Build history of the part. All positions in model axes, mm. A direction names the side the tool comes from. Coordinates: 2 decimals unless noted, no trailing zeros. Write each loop counter-clockwise with the first axis right and the second up, starting at its lowest first coordinate (ties: lowest second). Pieces come first, ordered by that corner, then holes.
```python
from build123d import *

# Parameters (mm, degrees)
SKETCH_1_W             = 130
SKETCH_1_H             = 130
EXTRUDE_1251_DEPTH     = 5
EXTRUDE_1478_DEPTH     = 25
SKETCH_3_R             = 17.5
CUT_EXTRUDE_1_DEPTH    = 85
SKETCH_4_R             = 17.5
CUT_EXTRUDE_2_DEPTH    = 85
SKETCH_8_W             = 52
SKETCH_8_H             = 25
CUT_EXTRUDE_1_2_DEPTH  = 10
SKETCH_9_W             = 52
SKETCH_9_H             = 25
CUT_EXTRUDE_2_2_DEPTH  = 10
SKETCH_5_W             = 2
SKETCH_5_H             = 2
SKETCH_5_H_2           = 43
SKETCH_5_W_2           = 43
EXTRUDE_2758_DEPTH     = 25
SKETCH_7_W             = 33.5
SKETCH_7_H             = 33.5
EXTRUDE_2892_DEPTH     = 13
HOLE_WIZARD_2949_D     = 5
HOLE_WIZARD_2949_DEPTH = 5
HOLE_WIZARD_2949_TIP   = 1.502151548
HOLE_WIZARD_1_D        = 2.5
HOLE_WIZARD_2_D        = 2.5
HOLE_WIZARD_6774_D     = 2.5
HOLE_WIZARD_1_2_D      = 2.5
HOLE_WIZARD_2_2_D      = 2.5


with BuildPart() as part:
    # 草图1 → Extrude 1251 (new body)
    with BuildSketch(Plane(origin=(0, 0, 0), x_dir=(1, 0, 0), z_dir=(0, 1, 0))):
        with Locations((65, 65)):
            Rectangle(SKETCH_1_W, SKETCH_1_H)
    extrude(amount=EXTRUDE_1251_DEPTH)

    # 草图2 → Extrude 1478 (add)
    with BuildSketch(Plane(origin=(0, 5, 0), x_dir=(1, 0, 0), z_dir=(0, 1, 0))):
        Polygon((0, 85), (0, 0), (52, 0), (52, 78), (130, 78), (130, 130), (45, 130), (45, 85), align=None)
    extrude(amount=EXTRUDE_1478_DEPTH)

    # 草图3 → Cut-Extrude 1 (cut)
    with BuildSketch(Plane.XY):
        with Locations((26.027680942, 22.5)):
            Circle(SKETCH_3_R)
    extrude(amount=-CUT_EXTRUDE_1_DEPTH, mode=Mode.SUBTRACT)

    # 草图4 → Cut-Extrude 2 (cut)
    with BuildSketch(Plane(origin=(130, 0, 0), x_dir=(0, 0, -1), z_dir=(1, 0, 0))):
        with Locations((104, 22.5)):
            Circle(SKETCH_4_R)
    extrude(amount=-CUT_EXTRUDE_2_DEPTH, mode=Mode.SUBTRACT)

    # 草图8 → Cut-Extrude 1 2 (cut)
    with BuildSketch(Plane(origin=(130, 0, 0), x_dir=(0, 0, -1), z_dir=(1, 0, 0))):
        with Locations((104, 17.5)):
            Rectangle(SKETCH_8_W, SKETCH_8_H)
    extrude(amount=-CUT_EXTRUDE_1_2_DEPTH, mode=Mode.SUBTRACT)

    # 草图9 → Cut-Extrude 2 2 (cut)
    with BuildSketch(Plane.XY):
        with Locations((26, 17.5)):
            Rectangle(SKETCH_9_W, SKETCH_9_H)
    extrude(amount=-CUT_EXTRUDE_2_2_DEPTH, mode=Mode.SUBTRACT)

    # 草图5 → Extrude 2758 (add)
    with BuildSketch(Plane(origin=(0, 5, 0), x_dir=(1, 0, 0), z_dir=(0, 1, 0))):
        with Locations((1, 129)):
            Rectangle(SKETCH_5_W, SKETCH_5_H)
        with Locations((1, 106.5)):
            Rectangle(SKETCH_5_W, SKETCH_5_H_2)
        with Locations((23.5, 129)):
            Rectangle(SKETCH_5_W_2, SKETCH_5_H)
    extrude(amount=EXTRUDE_2758_DEPTH)

    # 草图7 → Extrude 2892 (add)
    with BuildSketch(Plane(origin=(0, 5, 0), x_dir=(1, 0, 0), z_dir=(0, 1, 0))):
        with Locations((18.75, 111.25)):
            Rectangle(SKETCH_7_W, SKETCH_7_H)
    extrude(amount=EXTRUDE_2892_DEPTH)

    # Hole Wizard 2949
    with Locations(Plane(origin=(48, 0, -82), x_dir=(0, 0, -1), z_dir=(0, -1, 0))):
        with Locations((0, 0), (-25, 25)):
            Hole(HOLE_WIZARD_2949_D / 2, depth=HOLE_WIZARD_2949_DEPTH)
            with Locations((0, 0, -(HOLE_WIZARD_2949_DEPTH + HOLE_WIZARD_2949_TIP / 2))):  # 118° drill point
                Cone(0, HOLE_WIZARD_2949_D / 2, HOLE_WIZARD_2949_TIP, mode=Mode.SUBTRACT)

    # Hole Wizard 1 (through all)
    with Locations(Plane(origin=(0, 0, 0), x_dir=(-1, 0, 0), z_dir=(0, -1, 0))):
        with Locations((-26, 64), (-26, 79), (-26, 44), (-26, 24), (-26, 4)):
            Hole(HOLE_WIZARD_1_D / 2)

    # Hole Wizard 2 (through all)
    with Locations(Plane(origin=(0, 0, 0), x_dir=(-1, 0, 0), z_dir=(0, -1, 0))):
        with Locations((-66, 104), (-51, 104), (-86, 104), (-106, 104), (-126, 104)):
            Hole(HOLE_WIZARD_2_D / 2)

    # Hole Wizard 6774 (through all)
    with Locations(Plane(origin=(0, 18, 0), x_dir=(1, 0, 0), z_dir=(0, 1, 0))):
        with Locations((21.341257188, 121.386664873), (8.613335127, 108.658742812), (26, 104)):
            Hole(HOLE_WIZARD_6774_D / 2)

    # Hole Wizard 1 2 (through all)
    with Locations(Plane(origin=(52, 0, 0), x_dir=(0, 0, -1), z_dir=(1, 0, 0))):
        with Locations((44, 22.5), (24, 22.5), (64, 22.5)):
            Hole(HOLE_WIZARD_1_2_D / 2)

    # Hole Wizard 2 2 (through all)
    with Locations(Plane.XY.offset(-78)):
        with Locations((86, 22.5), (106, 22.5), (66, 22.5)):
            Hole(HOLE_WIZARD_2_2_D / 2)


solid = part.part
```
1. Flat gauge pins, fed straight in: pin 1 (8 mm diameter, centred on x = 106, z = -53, fed in from +Y); pin 2 (3 mm diameter, centred on x = 96.5, y = 12, fed in from +Z); pin 3 (1.5 mm diameter, centred on x = 26, z = -24, fed in from -Y); pin 4 (1.5 mm diameter, centred on y = 19, z = -28.5, fed in from +X). Where does each tip first touch, or does it go through?
Computed values:
pin 1: stops at y = 5
pin 2: stops at z = -78
pin 3: passes through
pin 4: stops at x = 52
2. Mould opens along Z. For faces 4 (the face through (47, 15, -10)), 5 (the face through (0, 15, -66)), 6 (the face through (45, 13, -89)) say: +Z half, -Z half, draft (parallel to the pull), parting line (faces both ways), or undercut.
Computed values:
face 4: +Z half
face 5: draft
face 6: undercut
3. 3-axis set-ups, long thin cutter, end or side, ignore diameter. For faces 1 (the face through (19, 11, -94.5)), 2 (the face through (52, 17, -44)), 3 (the face through (120, 15, -125)): which of +Z, -Z, +X, -X, +Y, -Y reach the whole face in a straight line?
Computed values:
face 1: +Y
face 2: +Z, +X, +Y
face 3: +Z, -Z, +X, +Y
4. Saw through at C-C on y = 27. List the corners of the cut face in (x, z).
Computed values:
outline: (0, -130) - (120, -130) - (120, -120.91) - (45, -120.91) - (45, -128) - (2, -128) - (2, -85) - (9.12, -85) - (9.12, -10) - (0, -10) - close; (42.94, -85) - (45, -85) - (45, -87.09) - (120, -87.09) - (120, -78) - (52, -78) - (52, -10) - (42.94, -10) - close
5. Saw through at A-A on y = 11. List the corners of the cut face in (x, z), plus the area to 3 significant figures.
Computed values:
outline: (0, -130) - (120, -130) - (120, -117.19) - (45, -117.19) - (45, -128) - (35.5, -128) - (35.5, -94.5) - (2, -94.5) - (2, -85) - (12.84, -85) - (12.84, -10) - (0, -10) - close; (39.22, -85) - (45, -85) - (45, -90.81) - (120, -90.81) - (120, -78) - (52, -78) - (52, -10) - (39.22, -10) - close; hole circle Ø2.5 at (8.61, -108.66); hole circle Ø2.5 at (21.34, -121.39); hole circle Ø2.5 at (26, -104)
area: 5,080 mm2
6. Probe line 1 along Z through (x, y) = (92.5, 23); line 2 along Z through (x, y) = (3, 22); line 3 along Z through (x, y) = (9, 7.5). List the from-to ranges inside material, lowest first.
Computed values:
line 1: z = -130 to -121.49, -86.51 to -78
line 2: z = -130 to -128, -85 to -65.15, -62.85 to -45.15, -42.85 to -25.15, -22.85 to -10
line 3: z = -130 to -109.85, -107.47 to -94.5, -85 to -10
7. Saw through at B-B on z = -57. List the corners of the cut face in (x, y), plus the area to 3 significant figures.
Computed values:
outline: (0, 0) - (70.5, 0) - (70.5, 5) - (52, 5) - (52, 30) - (41.84, 30) arc R17.5 cw (long way) to (10.22, 30) - (0, 30) - close; (75.5, 0) - (130, 0) - (130, 5) - (75.5, 5) - close
area: 1,190 mm2
8. Saw through at D-D on x = 57.5. List the corners of the cut face in (y, z).
Computed values:
outline: (0, -130) - (30, -130) - (30, -119.81) arc R17.5 cw (long way) to (30, -88.19) - (30, -78) - (5, -78) - (5, 0) - (0, 0) - close
